Autodesk Inventor part; units mm, degrees
ref_plane "YZ Plane" through (0, 0, 0) normal (1, 0, 0) x (0, 1, 0)
ref_plane "XZ Plane" through (0, 0, 0) normal (0, 1, 0) x (-1, 0, 0)
ref_plane "XY Plane" through (0, 0, 0) normal (0, 0, 1) x (1, 0, 0)
sketch "스케치1" plane through (0, 0, 0) normal (0, 1, 0) x (-1, 0, 0)
  line L0 (0, 0) -> (-45.2, 0)
  line L1 (-45.2, 0) -> (-45.2, -15.1)
  line L2 (-45.2, -15.1) -> (0, -15.1)
  line L3 (0, -15.1) -> (0, 0)
  dimension "d0" = 45.2
  dimension "d1" = 15.1
extrude "돌출1" add sketch "스케치1" along normal blind 3.7
sketch "스케치2" plane through (0, 3.7, 0) normal (0, 1, 0) x (1, 0, 0)
  line L0 (0, 0) -> (45.2, 0)
  line L1 (45.2, 15.1) -> (0, 15.1)
  line L2 (0, 0) -> (4.4, 0)
  line L3 (4.4, 0) -> (4.4, 15.1)
  line L4 (4.4, 15.1) -> (0, 15.1)
  line L5 (0, 15.1) -> (0, 0)
  line L6 (4.4, 15.1) -> (14.4, 15.1)
  line L7 (14.4, 15.1) -> (14.4, 0)
  line L8 (14.4, 0) -> (4.4, 0)
  line L9 (4.4, 0) -> (4.4, 15.1)
  line L10 (14.4, 0) -> (13.4, 0)
  line L11 (13.4, 0) -> (15.4, 0)
  line L12 (13.4, 0) -> (5.6, 0)
  line L13 (5.6, 0) -> (5.6, 15.1)
  line L14 (5.6, 15.1) -> (13.4, 15.1)
  line L15 (13.4, 15.1) -> (13.4, 0)
  line L16 (15.4, 0) -> (23.2, 0)
  line L17 (23.2, 0) -> (23.2, 15.1)
  line L18 (23.2, 15.1) -> (15.4, 15.1)
  line L19 (15.4, 15.1) -> (15.4, 0)
  line L20 (23.2, 15.1) -> (45.2, 15.1)
  line L21 (45.2, 15.1) -> (45.2, 0)
  line L22 (45.2, 0) -> (23.2, 0)
  line L23 (23.2, 0) -> (23.2, 15.1)
  dimension "d4" = 4.4
  dimension "d5" = 10
  dimension "d6" = 1
  dimension "d7" = 2
  dimension "d8" = 7.8
  dimension "d9" = 7.8
extrude "돌출2" cut sketch "스케치2" against normal blind 2.5 contours L5 L1 L3 L0 | L15 L1 L7 L0 | L7 L1 L19 L0 | L17 L1 L21 L0
offset faces "크기1" outward -0.75 faces at (13.4, 2.8667, -10.0667) (15.4, 2.8667, -5.0333)
offset faces "크기2" outward 1.2 faces at (23.2, 2.0333, -5.0333)
properties part number "BMS"
Can you work these out from the model? Positions are in its coordinate system, mm. A direction names the side the tool comes from. Give positions to 0.01 mm unless a question says otherwise; leave off trailing zeros. Loops run counter-clockwise (first coordinate to the right, second up) from the corner with the lowest first, then second, coordinate; pieces in that order, holes last. Notation, with made-up numbers: (-23.75, 79) - (-18.75, 79) arc R10 ccw to (-18.75, 83) - close; hole circle Ø1 at (-40, 43.25). An arc over 180 degrees is marked (long way). Return JSON: item names as keys, results as strings.
1. I want a section at A-A on y = 3. Please give me the cut outline in (x, z), and give its area (3 significant figures).
Output values:
{"outline": "(4.4, -15.1) - (12.65, -15.1) - (12.65, 0) - (4.4, 0) - close; (16.15, -15.1) - (24.4, -15.1) - (24.4, 0) - (16.15, 0) - close", "area": "249 mm²"}
2. I want a section at B-B on z = -4. Please give me the cut outline in (x, y).
Output values:
{"outline": "(0, 0) - (45.2, 0) - (45.2, 1.2) - (24.4, 1.2) - (24.4, 3.7) - (16.15, 3.7) - (16.15, 1.2) - (12.65, 1.2) - (12.65, 3.7) - (4.4, 3.7) - (4.4, 1.2) - (0, 1.2) - close"}
3. We'd pull the mould along X, two halves only. Please class faces 1 (the face through (2, 1.2, -8)), 2 (the face through (24.4, 2, -7)), 3 (the face through (14, 1.2, -8)): +X half, -X half, draft (parallel to the pull), parting line (faces both ways), or undercut.
Output values:
{"face 1": "draft", "face 2": "+X half", "face 3": "undercut"}
4. I'm going to push flat-ended pins straight in: pin 1 Ø1.2 at (y, z) = (2.5, -6) entering from +X; pin 2 Ø0.8 at (y, z) = (2, -10) entering from -X; pin 3 Ø1 at (x, z) = (14.5, -8.5) entering from +Y. Where does each tip first touch, or does it pass through?
Output values:
{"pin 1": "stops at x = 24.4", "pin 2": "stops at x = 4.4", "pin 3": "stops at y = 1.2"}
5. If I drill on line 1 (X direction, y = 1.65, z = -12); line 2 (Y direction, x = 3.5, z = -8.75), over which ranges is the centre line in solid material (lowest first)?
Output values:
{"line 1": "x = 4.4 to 12.65, 16.15 to 24.4", "line 2": "y = 0 to 1.2"}
6. I want a section at C-C on x = 25. Please give me the cut outline in (y, z).
Output values:
{"outline": "(0, -15.1) - (1.2, -15.1) - (1.2, 0) - (0, 0) - close"}
7. For faces 4 (the face through (35, 1.2, -8)), 5 (the face through (4.4, 2, -7)), 6 (the face through (16.15, 2, -8)), 7 (the face through (20, 3.7, -7)), which set-ups out of +Z, -Z, +X, -X, +Y, -Y let a thin tool reach every point of the face, with its end or its side?
Output values:
{"face 4": "+Z, -Z, +X, +Y", "face 5": "+Z, -Z, -X, +Y", "face 6": "+Z, -Z, +Y", "face 7": "+Z, -Z, +X, -X, +Y"}
